Study the drawing (mm; zero at the part's minimum x, y, z) and answer. A direction names the side the tool comes from. Give positions to 0.01 mm unless a question says otherwise; leave off trailing zeros. Order: outer loops, then holes, each group sorted by start corner. A loop starts at its lowest first (then second) coordinate and runs counter-clockwise, first axis right, second up.
Item 1: Find the intervals of material crossed by line 1 along X through (y, z) = (13, 45); line 2 along Z through (x, y) = (50, 8.75); line 3 along Y through (x, z) = (53, 24.5), in increasing order.
Item 2: A cutting plane is placed at B-B (y = 6.5). Write down the section's boundary in (x, z) (1 decimal), plus the area to 3 significant figures.
Item 3: Given pin 1 Ø5 at (y, z) = (10.5, 25) entering from +X; pin 2 Ø1 at (x, y) = (10, 32) entering from +Z; pin 3 Ø3 at (x, z) = (50, 45) entering from +Y; pin 4 Ø13.5 at (y, z) = (9.5, 37.5) entering from -X, each flat-ended and moving along its own axis, determine where each tip first touches the part or whether it passes through.
Item 4: A cutting plane is placed at A-A (z = 45). Write down the section's boundary in (x, y), plus the area to 3 significant figures.
Item 5: A cutting plane is placed at C-C (x = 48.5). Write down the section's boundary in (y, z).
Item 6: A cutting plane is placed at D-D (x = 29.5). Write down the section's boundary in (y, z).
Item 7: Which of the six approach directions +Z, -Z, +X, -X, +Y, -Y give full straight-line access (tool end or side, diameter ignored) to the marked faces 1, 2, 3 and 4?
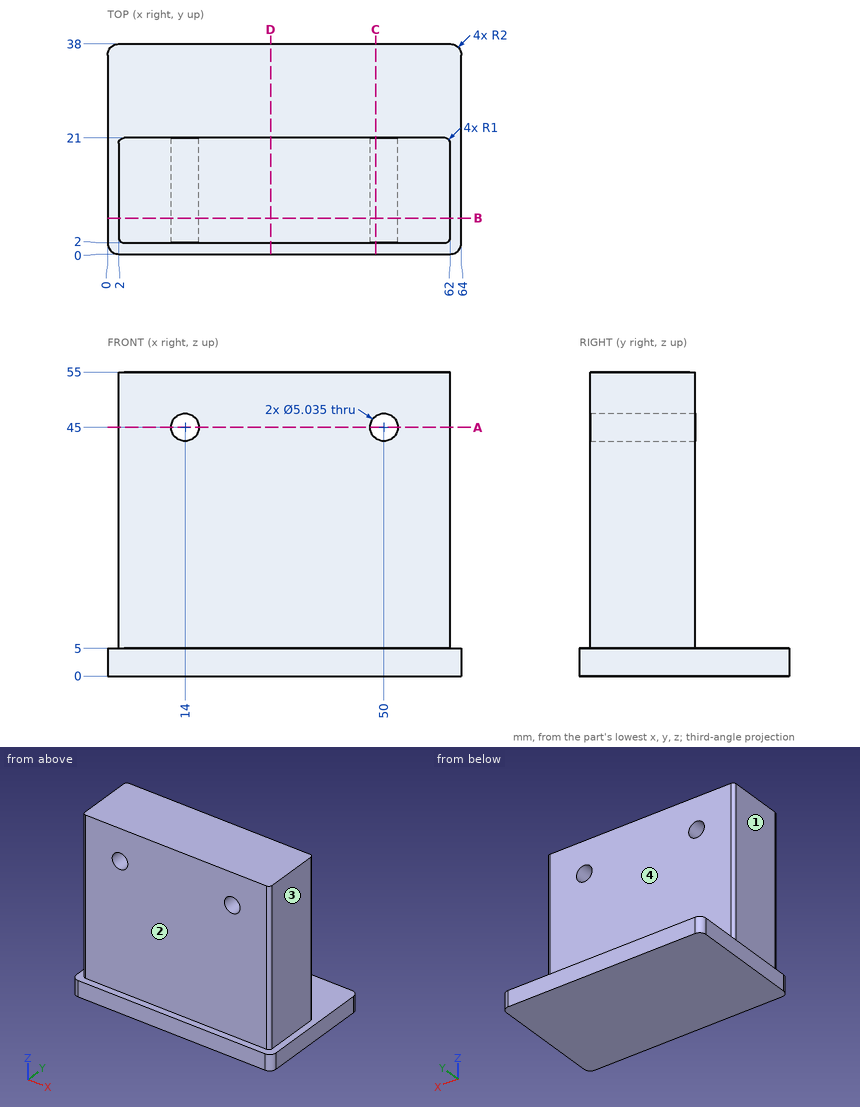
Response values:
1. line 1: x = 2 to 11.48, 16.52 to 47.48, 52.52 to 62
1. line 2: z = 0 to 42.48, 47.52 to 55
1. line 3: y = 2 to 21
2. outline: (0, 0) - (64, 0) - (64, 5) - (62, 5) - (62, 55) - (2, 55) - (2, 5) - (0, 5) - close; hole circle Ø5 at (14, 45); hole circle Ø5 at (50, 45)
2. area: 3,280 mm2
3. pin 1: stops at x = 62
3. pin 2: stops at z = 5
3. pin 3: passes through
3. pin 4: stops at x = 2
4. outline: (2, 3) arc R1 ccw to (3, 2) - (11.48, 2) - (11.48, 21) - (3, 21) arc R1 ccw to (2, 20) - close; (16.52, 2) - (47.48, 2) - (47.48, 21) - (16.52, 21) - close; (52.52, 2) - (61, 2) arc R1 ccw to (62, 3) - (62, 20) arc R1 ccw to (61, 21) - (52.52, 21) - close
4. area: 948 mm2
5. outline: (0, 0) - (38, 0) - (38, 5) - (21, 5) - (21, 42.98) - (2, 42.98) - (2, 5) - (0, 5) - close; (2, 47.02) - (21, 47.02) - (21, 55) - (2, 55) - close
6. outline: (0, 0) - (38, 0) - (38, 5) - (21, 5) - (21, 55) - (2, 55) - (2, 5) - (0, 5) - close
7. face 1: +Z, -X, +Y, -Y
7. face 2: +Z, +X, -X, -Y
7. face 3: +Z, +X, +Y, -Y
7. face 4: +Z, +X, -X, +Y
